Input: part model. Units: mm. Frame: model coordinates. Face numbers are marked on the shaded views. A direction names the side the tool comes from. Give positions to 0.01 mm unless a question says otherwise; leave off trailing zeros. Loops run counter-clockwise (first coordinate to the right, second up) from the corner with the lowest first, then second, coordinate; pieces in that order, holes last. Notation, with made-up numbers: M 38,32.25 L 44,32.25 A21 cw 44,61.25 Z; hole C 25.25,54.5 d3. An arc over 180 degrees is marked long. Answer as a JSON object with one key per item and string values. Group by question number.
```python
from build123d import *

# Parameters (mm, degrees)
SKETCH1_W               = 105
SKETCH1_H               = 75
BOSS_EXTRUDE1_DEPTH     = 80
SHELL1_T                = -10
SKETCH2_W               = 10
SKETCH2_H               = 60
BOSS_EXTRUDE2_DEPTH     = 60
FILLET1_R               = 5
SKETCH3_W               = 75
SKETCH3_H               = 50
CUT_EXTRUDE1_DEPTH      = 152.822264507
SKETCH4_W               = 55
SKETCH4_H               = 40
CUT_EXTRUDE2_DEPTH      = 152.822264507
SKETCH5_W               = 15
SKETCH5_H               = 7.5
BOSS_EXTRUDE3_DEPTH     = 20
SKETCH6_R               = 4
CUT_EXTRUDE3_DEPTH      = 163.807401552
MIRROR2_COPY_1_SKETCH_W = 15
MIRROR2_COPY_1_SKETCH_H = 7.5
MIRROR2_COPY_1_DEPTH    = 20
MIRROR2_COPY_2_SKETCH_R = 4
MIRROR2_COPY_2_DEPTH    = 163.807401552
FILLET3_R               = 2
SKETCH7_W               = 29
SKETCH7_H               = 6
CUT_EXTRUDE4_DEPTH      = 15
SKETCH8_W               = 29
SKETCH8_H               = 6
BOSS_EXTRUDE4_DEPTH     = 35
SKETCH9_R               = 4.2
CUT_EXTRUDE5_DEPTH      = 35


with BuildPart() as part:
    # Sketch1 → Boss-Extrude1 (new body)
    with BuildSketch(Plane(origin=(0, 0, 0), x_dir=(1, 0, 0), z_dir=(0, 1, 0))):
        with Locations((52.5, 37.5)):
            Rectangle(SKETCH1_W, SKETCH1_H)
    extrude(amount=BOSS_EXTRUDE1_DEPTH)

    # Shell1
    shell1_openings = [part.faces().sort_by_distance(p)[0] for p in [
        (0, 40, -37.5),
    ]]
    offset(amount=SHELL1_T, openings=shell1_openings, kind=Kind.INTERSECTION)

    # Sketch2 → Boss-Extrude2 (add)
    with BuildSketch(Plane.XY.offset(-65)):
        with Locations((5, 40)):
            Rectangle(SKETCH2_W, SKETCH2_H)
    extrude(amount=BOSS_EXTRUDE2_DEPTH)

    # Fillet1
    fillet1_edges = [part.edges().sort_by_distance(p)[0] for p in [
        (105, 80, -37.5),
        (52.5, 80, -75),
        (0, 80, -37.5),
        (52.5, 0, -75),
        (105, 0, -37.5),
        (52.5, 0, 0),
        (0, 0, -37.5),
        (52.5, 80, 0),
    ]]
    fillet(fillet1_edges, radius=FILLET1_R)

    # Sketch3 → Cut-Extrude1 (cut, through all)
    with BuildSketch(Plane.XY):
        with Locations((52.5, 40)):
            Rectangle(SKETCH3_W, SKETCH3_H)
    extrude(amount=-CUT_EXTRUDE1_DEPTH, mode=Mode.SUBTRACT)

    # Sketch4 → Cut-Extrude2 (cut, through all)
    with BuildSketch(Plane.ZY):
        with Locations((-37.5, 40)):
            Rectangle(SKETCH4_W, SKETCH4_H)
    extrude(amount=-CUT_EXTRUDE2_DEPTH, mode=Mode.SUBTRACT)

    # Sketch5 → Boss-Extrude3 (add)
    with BuildSketch(Plane(origin=(105, 0, 0), x_dir=(0, 0, -1), z_dir=(1, 0, 0))):
        with Locations((22.5, 68.75)):
            Rectangle(SKETCH5_W, SKETCH5_H)
    boss_extrude3 = extrude(amount=BOSS_EXTRUDE3_DEPTH)

    # Sketch6 → Cut-Extrude3 (cut, through all)
    with BuildSketch(Plane(origin=(0, 72.5, 0), x_dir=(1, 0, 0), z_dir=(0, 1, 0))):
        with BuildLine():
            Line((125, 30), (120, 30))
            ThreePointArc((120, 30), (123.535533906, 28.535533906), (125, 25))
            Line((125, 25), (125, 30))
        make_face()
        with Locations(Location((116.877501001, 22.5, 0), (0, 0, 270))):
            Circle(SKETCH6_R)
        with BuildLine():
            ThreePointArc((125, 20), (123.535533906, 16.464466094), (120, 15))
            Line((120, 15), (125, 15))
            Line((125, 15), (125, 20))
        make_face()
    cut_extrude3 = extrude(amount=-CUT_EXTRUDE3_DEPTH, mode=Mode.SUBTRACT)

    # Mirror1: Boss-Extrude3, Cut-Extrude3 across plane
    add(boss_extrude3.mirror(Plane(origin=(52.5, 0, 0), x_dir=(0, 0, 1), z_dir=(1, 0, 0))))
    add(cut_extrude3.mirror(Plane(origin=(52.5, 0, 0), x_dir=(0, 0, 1), z_dir=(1, 0, 0))), mode=Mode.SUBTRACT)

    # Mirror2: Boss-Extrude3, Cut-Extrude3 across plane
    add(boss_extrude3.mirror(Plane.XY.offset(-37.5)))
    add(cut_extrude3.mirror(Plane.XY.offset(-37.5)), mode=Mode.SUBTRACT)

    # Mirror2 copy 1 sketch → Mirror2 copy 1 (add)
    with BuildSketch(Plane(origin=(0, 0, -75), x_dir=(0, 0, 1), z_dir=(-1, 0, 0))):
        with Locations((22.5, 68.75)):
            Rectangle(MIRROR2_COPY_1_SKETCH_W, MIRROR2_COPY_1_SKETCH_H)
    extrude(amount=MIRROR2_COPY_1_DEPTH)

    # Mirror2 copy 2 sketch → Mirror2 copy 2 (cut, through all)
    with BuildSketch(Plane(origin=(105, 72.5, -75), x_dir=(-1, 0, 0), z_dir=(0, 1, 0))):
        with BuildLine():
            Line((125, 30), (120, 30))
            ThreePointArc((120, 30), (123.535533906, 28.535533906), (125, 25))
            Line((125, 25), (125, 30))
        make_face()
        with Locations(Location((116.877501001, 22.5, 0), (0, 0, 270))):
            Circle(MIRROR2_COPY_2_SKETCH_R)
        with BuildLine():
            ThreePointArc((125, 20), (123.535533906, 16.464466094), (120, 15))
            Line((120, 15), (125, 15))
            Line((125, 15), (125, 20))
        make_face()
    extrude(amount=-MIRROR2_COPY_2_DEPTH, mode=Mode.SUBTRACT)

    # Fillet3
    fillet3_edges = [part.edges().sort_by_distance(p)[0] for p in [
        (105, 68.75, -15),
        (105, 65, -22.5),
        (105, 68.75, -30),
        (105, 72.5, -22.5),
        (0, 68.75, -15),
        (0, 65, -22.5),
        (0, 68.75, -30),
        (0, 72.5, -22.5),
        (0, 68.75, -60),
        (0, 65, -52.5),
        (0, 68.75, -45),
        (0, 72.5, -52.5),
        (105, 68.75, -60),
        (105, 65, -52.5),
        (105, 68.75, -45),
        (105, 72.5, -52.5),
    ]]
    fillet(fillet3_edges, radius=FILLET3_R)

    # Sketch7 → Cut-Extrude4 (cut)
    with BuildSketch(Plane(origin=(0, 80, 0), x_dir=(1, 0, 0), z_dir=(0, 1, 0))):
        with Locations((52.5, 37.5)):
            Rectangle(SKETCH7_W, SKETCH7_H)
    extrude(amount=-CUT_EXTRUDE4_DEPTH, mode=Mode.SUBTRACT)

    # Sketch8 → Boss-Extrude4 (add)
    with BuildSketch(Plane(origin=(0, 80, 0), x_dir=(1, 0, 0), z_dir=(0, 1, 0))):
        with Locations((52.5, 46.877224158)):
            Rectangle(SKETCH8_W, SKETCH8_H)
        with Locations((52.5, 27.56334528)):
            Rectangle(SKETCH8_W, SKETCH8_H)
    extrude(amount=BOSS_EXTRUDE4_DEPTH)

    # Sketch9 → Cut-Extrude5 (cut)
    with BuildSketch(Plane.XY.offset(-24.56334528)):
        with BuildLine():
            Line((38, 115), (38, 97.5))
            Line((38, 97.5), (48.649892195, 110.353318167))
            ThreePointArc((48.649892195, 110.353318167), (52.5, 112.163228843), (56.350107805, 110.353318167))
            Line((56.350107805, 110.353318167), (67, 97.5))
            Line((67, 97.5), (67, 115))
            Line((67, 115), (38, 115))
        make_face()
        with Locations((52.5, 91)):
            Circle(SKETCH9_R)
    extrude(amount=-CUT_EXTRUDE5_DEPTH, mode=Mode.SUBTRACT)


solid = part.part
```
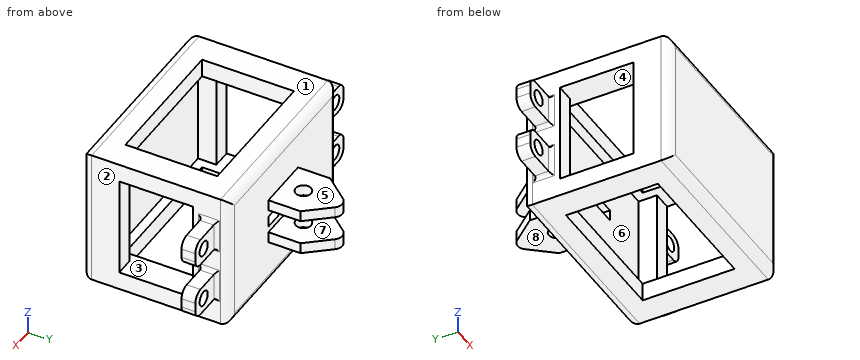
1. First-contact query: P1, Ø5, axis at y = 77.5, z = -37.5, coming from the +X side; P2, Ø1.5, axis at y = 85.5, z = -44.5, coming from the -X side; P3, Ø9, axis at x = 116.88, z = -22.5, coming from the +Y side; P4, Ø3, axis at x = 63.5, y = 68, coming from the +Z side. Flat tips, straight axial feed; report the tip coordinate or a pass-through.
2. Section C-C (x = 115). Output: boundary loops of the cut face in (y, z), then the cut area to 3 significant figures.
3. Section B-B (y = 91). Output: boundary loops of the cut face in (x, z), then the cut area to 3 significant figures.
4. Section A-A (x = 76.5). Output: boundary loops of the cut face in (y, z), then the cut area to 3 significant figures.
5. Section D-D (z = -52.5). Count the separate pieces of the cut face and the enclosed holes in it, then the cut area to 3 significant figures.
6. Material intervals for L1, parallel to Y at x = 52.5, z = -27.6; L2, parallel to X at y = 69, z = -52; L3, parallel to X at y = 70.25, z = -22.5, sorted ascending.
7. Reachability of the marked faces 5, 6, 7 and 8 from +Z, -Z, +X, -X, +Y, -Y: full face, straight path, thin tool, end or side. Return the list, or none.
8. Mould query, pull axis X, two halves, no side actions, for the marked faces 1, 2, 3 and 4. Classes: pulls with the +X half, pulls with the -X half, needs draft (parallel to the pull), parting line crosses it, or undercut.
Geometry results:
{
 "1": {"P1": "x = 105", "P2": "x = 38", "P3": "y = 72.5", "P4": "z = 0"},
 "2": {"outline": "M 65,-60 L 72.5,-60 L 72.5,-56.03 L 65,-56.03 Z; M 65,-48.97 L 72.5,-48.97 L 72.5,-45 L 65,-45 Z; M 65,-30 L 72.5,-30 L 72.5,-26.03 L 65,-26.03 Z; M 65,-18.97 L 72.5,-18.97 L 72.5,-15 L 65,-15 Z", "area": "119 mm2"},
 "3": {"outline": "M 38,-49.88 L 48.3,-49.88 L 48.3,-43.88 L 38,-43.88 Z; M 38,-30.56 L 48.3,-30.56 L 48.3,-24.56 L 38,-24.56 Z; M 56.7,-49.88 L 67,-49.88 L 67,-43.88 L 56.7,-43.88 Z; M 56.7,-30.56 L 67,-30.56 L 67,-24.56 L 56.7,-24.56 Z", "area": "247 mm2"},
 "4": {"outline": "M 0,-70 A5 ccw 5,-75 L 15,-75 L 15,-65 L 10,-65 L 10,-10 L 15,-10 L 15,0 L 5,0 A5 ccw 0,-5 Z; M 65,-75 L 75,-75 A5 ccw 80,-70 L 80,-5 A5 ccw 75,0 L 65,0 L 65,-10 L 70,-10 L 70,-65 L 65,-65 Z", "area": "1,680 mm2"},
 "5": {"separate pieces": "4", "enclosed holes": "0", "area": "2,660 mm2"},
 "6": {"L1": "0 to 10, 70 to 86.8, 95.2 to 112.16", "L2": "-20 to -15.85, -7.91 to 10, 95 to 112.91, 120.85 to 125", "L3": "-20 to -15.88, -7.88 to 112.88, 120.88 to 125"},
 "7": {"face 5": "+Z, +X, -X, +Y", "face 6": "none", "face 7": "+X, -X, +Y", "face 8": "-Z, +X, -X, +Y"},
 "8": {"face 1": "needs draft", "face 2": "pulls with the +X half", "face 3": "undercut", "face 4": "undercut"}
}
